Check sheet for the modelled part. Datum: model origin and axes. Units: mm. Round coordinates to 2 decimals unless told otherwise and drop trailing zeros. Write each loop counter-clockwise with the first axis right and the second up, starting at its lowest first coordinate (ties: lowest second). Pieces come first, ordered by that corner, then holes. Notation, with made-up numbers: M 66.5,-6 L 76.5,-6 A25 ccw 76.5,13 Z; hole C 68,81 d8. An arc over 180 degrees is marked long. One line per item, written item: value.
from build123d import *

# Parameters (mm, degrees)
SKETCH2_R = 0.8


with BuildPart() as part:
    # Sweep1: sweep along a path in Sketch1
    with BuildLine(Plane.XY) as sweep1_path:
        Line((-7.5, 54.2), (-7.5, 24.158431222))
        ThreePointArc((-7.5, 24.158431222), (-8.283629786, 21.471011972), (-10.388888889, 19.625969432))
        ThreePointArc((-10.388888889, 19.625969432), (-12.073096171, 18.1499354), (-12.7, 16))
        Line((-12.7, 16), (-12.7, 0))
    # Sketch2 → Sweep1 (sweep)
    with BuildSketch(Plane(origin=(0, 0, 0), x_dir=(1, 0, 0), z_dir=(0, 1, 0))):
        with Locations((-12.7, 0)):
            Circle(SKETCH2_R)
    sweep(path=sweep1_path.line)

    # Sketch3 → Revolve1 (revolve)
    with BuildSketch(Plane.XY):
        with BuildLine():
            Line((-12.7, 0), (-11.7, 0))
            Line((-11.7, 0), (-11.7, 16))
            ThreePointArc((-11.7, 16), (-11.734074174, 16.258819045), (-11.833974596, 16.5))
            Line((-11.833974596, 16.5), (-12.7, 18))
            Line((-12.7, 18), (-12.7, 0))
        make_face()
    revolve(axis=Axis((-12.7, 21.819423219, 0), (0, -1, 0)))


solid = part.part
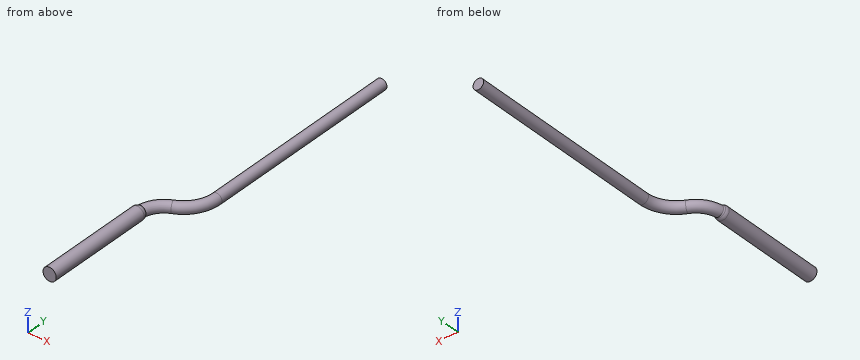
Q1. Scan lines: line 1 (Z direction, x = -12.75, y = 15.5); line 2 (Y direction, x = -10.5, z = 0.2); line 3 (Y direction, x = -7.75, z = 0.55). Record each from-to range of solid material in increasing order. Write a range as [from, to].
Completed:
line 1: [-1, 1]
line 2: [18.68, 20.44]
line 3: [21.23, 54.2]
Q2. Sectioned sample at B-B on y = 50. Enter the section's corners in (x, z), and give its area (3 significant figures).
Completed:
outline: C -7.5,0 d1.6
area: 2.01 mm^2
Q3. Depth check by flat-ended pin: P1, Ø1, axis at y = 40, z = 0.5, coming from the -X side. Enter the tip coordinate at first touch or a pass-through.
Completed:
P1: x = -8.3
Q4. Sectioned sample at A-A on y = 13. Enter the section's corners in (x, z).
Completed:
outline: C -12.7,0 d2
